Read the model definition and answer for the solid it produces. Units are mm, in the model's axes. A direction names the side the tool comes from. Round coordinates to 2 decimals unless told otherwise and drop trailing zeros. Loops run counter-clockwise (first coordinate to the right, second up) from the corner with the lowest first, then second, coordinate; pieces in that order, holes last. Notation, with made-up numbers: M 32,67.25 L 90,67.25 A8 cw 90,81.25 Z; hole C -30,49.25 d10. An arc over 180 degrees is marked long. Write each question's results on one line, items separated by ' | '.
Autodesk Fusion 360 part; units mm, degrees
sketch "Sketch1" plane through (0, 0, 0) normal (0, 0, 1) x (1, 0, 0)
sketch "Sketch2" plane through (0, 0, 0) normal (0, 1, 0) x (1, 0, 0)
  circle A0 centre (0, 0) radius 25
  circle A1 centre (0, 0) radius 27
  line L0 (-55, 0) -> (55, 0)
  line L1 (-55, 0) -> (-55, 3)
  line L2 (-55, 3) -> (55, 3)
  line L3 (55, 0) -> (55, 3)
  dimension "d1" = 50
  dimension "d2" = 2
extrude "Extrude1" add sketch "Sketch2" along normal blind 18.166 contours A0 A1 L0 | A0 A1 L0 L2 | A0 A1 L0 L2 | A1 L0 L2 L3 | A1 L0 L1 L2
fillet "Fillet1" radius 3.06 2 edges at (-27, 9.083, 0) (27, 9.083, 0)
fillet "Fillet2" radius 2.455 2 edges at (-24.8193, 9.083, -3) (24.8193, 9.083, -3)
fillet "Fillet3" radius 1.852 4 edges at (-55, 0, -1.5) (-55, 18.166, -1.5) (55, 0, -1.5) (55, 18.166, -1.5)
hole "Hole1" at (42.4144, 9.083, 0) direction (0, 0, -1) diameter 5 depth 7 tip angle 118 countersink diameter 8 countersink angle 90
hole "Hole2" at (-42.4144, 9.083, 0) direction (0, 0, -1) diameter 5 depth 7 tip angle 118 countersink diameter 8 countersink angle 90
1. Determine the mould class of faces 4 (the face through (-44.893, 9.408, -2.26)), 5 (the face through (25.716, 9.21, -2.283)), 6 (the face through (54.472, 0.557, -1.521)), 7 (the face through (0.555, 8.956, 26.994)) for opening direction X: released by +X, released by -X, zero draft, split by the parting line, or undercut.
Completed:
face 4: undercut | face 5: undercut | face 6: released by +X | face 7: split by the parting line
2. Find the intervals of material crossed by L1, parallel to Z at x = -37, y = 15.5; L2, parallel to X at y = 3.5, z = 9.25; L3, parallel to Z at x = 0, y = 3.5, in increasing order.
Completed:
L1: z = -3 to 0 | L2: x = -25.37 to -23.23, 23.23 to 25.37 | L3: z = 25 to 27
3. Given P1, Ø4.5, axis at x = -42.41, y = 9.08, coming from the -Z side; P2, Ø2, axis at y = 10, z = 7, coming from the +X side; P3, Ø2, axis at x = -30, y = 15.5, coming from the +Z side; P4, Ø8, axis at y = 3, z = 9, coming from the +X side, each flat-ended and moving along its own axis, determine where each tip first touches the part or whether it passes through.
Completed:
P1: passes through | P2: stops at x = 26.32 | P3: stops at z = 0.14 | P4: stops at x = 26.53
4. Which of the six approach directions +Z, -Z, +X, -X, +Y, -Y give full straight-line access (tool end or side, diameter ignored) to faces 1 (the face through (-42.6, 4.9, 0)), 2 (the face through (42.3, 4.9, 0)), 3 (the face through (-55, 9, -1))?
Completed:
face 1: +Z, -X, +Y, -Y | face 2: +Z, +X, +Y, -Y | face 3: +Z, -Z, -X, +Y, -Y
5. Find section B-B, the plane x = 0. Give the vertices of the cut face in (y, z).
Completed:
outline: M 0,25 L 18.17,25 L 18.17,27 L 0,27 Z
6. Find section C-C, the plane z = 20. Give the vertices of the cut face in (x, y).
Completed:
outline: M -18.14,0 L -15,0 L -15,18.17 L -18.14,18.17 Z; M 15,0 L 18.14,0 L 18.14,18.17 L 15,18.17 Z
7. Find section A-A, the plane z = 14.25. Give the vertices of the cut face in (x, y), then the cut area to 3 significant figures.
Completed:
outline: M -22.93,0 L -20.54,0 L -20.54,18.17 L -22.93,18.17 Z; M 20.54,0 L 22.93,0 L 22.93,18.17 L 20.54,18.17 Z | area: 86.9 mm2
